For this review, take the finished solid that the model builds, in its own axes (mm). A direction names the side the tool comes from. Give positions to 0.01 mm unless a question says otherwise; leave off trailing zeros. Loops run counter-clockwise (first coordinate to the right, second up) from the corner with the lowest first, then second, coordinate; pieces in that order, holes last. Notation, with made-up numbers: (82.5, -17.75) -> (132.5, -17.75) arc R30 cw to (132.5, 12.25) -> close; hole circle Ø11 at (46, 56.25). An arc over 180 degrees is marked (long way). Write each question's results on one line, items separated by ' | '. Start each with the question number.
```python
from build123d import *

# Parameters (mm, degrees)
SKETCH103_R           = 15
SKETCH103_R_2         = 8
PAD055_DEPTH          = 8.5
POCKET033_DEPTH       = 95.040009
POLARPATTERN024_COUNT = 4
POCKET034_DEPTH       = 2
POLARPATTERN025_COUNT = 4
SKETCH108_R           = 1
POCKET035_DEPTH       = 8.501


with BuildPart() as part:
    # Sketch103 → Pad055 (new body)
    with BuildSketch(Plane.YZ):
        Circle(SKETCH103_R)
        Circle(SKETCH103_R_2, mode=Mode.SUBTRACT)
    extrude(amount=-PAD055_DEPTH)

    # Sketch107 (on Face3 of Pad055) → Pocket033 (cut, through all)
    with BuildSketch(Plane.YZ):
        with BuildLine():
            ThreePointArc((4.120305, 6.857338), (6.382423, 7.966433), (4.442476, 9.573877))
            ThreePointArc((4.851745, 12.86394), (2.086453, 11.537443), (4.442476, 9.573877))
            ThreePointArc((12.86394, 4.851745), (9.721636, 9.721636), (4.851745, 12.86394))
            ThreePointArc((9.573874, 4.442468), (11.537447, 2.086454), (12.86394, 4.851745))
            ThreePointArc((9.573874, 4.442468), (7.966437, 6.382423), (6.857338, 4.120305))
            ThreePointArc((6.857338, 4.120305), (5.656854, 5.656854), (4.120305, 6.857338))
        make_face()
    pocket033 = extrude(amount=-POCKET033_DEPTH, mode=Mode.SUBTRACT)

    # PolarPattern024: Pocket033 ×4 about axis
    polarpattern024_axis = Axis((0, 0, 0), (1, 0, 0))
    for i in range(1, POLARPATTERN024_COUNT):
        add(pocket033.rotate(polarpattern024_axis, i * 360 / POLARPATTERN024_COUNT), mode=Mode.SUBTRACT)

    # Sketch105 (on ShapeBinder) → Pocket034 (cut)
    with BuildSketch(Plane(origin=(-8.5, 0, 0), x_dir=(0, -1, 0), z_dir=(-1, 0, 0))):
        with BuildLine():
            ThreePointArc((2.107476, 12.131304), (1.313608, 13.264776), (0, 13.7))
            Line((0, 13.7), (0, 0))
            Line((0, 0), (13.7, 0))
            ThreePointArc((13.7, 0), (13.264776, 1.313608), (12.131304, 2.107476))
            Line((7.14341, 3.601623), (12.131304, 2.107476))
            ThreePointArc((7.14341, 3.601623), (5.656854, 5.656854), (3.601623, 7.14341))
            Line((2.107476, 12.131304), (3.601623, 7.14341))
        make_face()
    pocket034 = extrude(amount=-POCKET034_DEPTH, mode=Mode.SUBTRACT)

    # PolarPattern025: Pocket034 ×4 about axis
    polarpattern025_axis = Axis((-8.5, 0, 0), (-1, 0, 0))
    for i in range(1, POLARPATTERN025_COUNT):
        add(pocket034.rotate(polarpattern025_axis, i * 360 / POLARPATTERN025_COUNT), mode=Mode.SUBTRACT)

    # Sketch108 (on ShapeBinder) → Pocket035 (cut, through all)
    with BuildSketch(Plane(origin=(-8.5, 0, 0), x_dir=(0, -1, 0), z_dir=(-1, 0, 0))):
        with Locations((0, 11.5)):
            Circle(SKETCH108_R)
        with Locations((11.5, 0)):
            Circle(SKETCH108_R)
        with Locations((0, -11.5)):
            Circle(SKETCH108_R)
        with Locations((-11.5, 0)):
            Circle(SKETCH108_R)
    extrude(amount=-POCKET035_DEPTH, mode=Mode.SUBTRACT)


with BuildPart() as part_1:
    # Body038 placement: moved
    add(part.part.moved(Location((18.5, 0, 0))))


solid = part_1.part
```
1. We need section A-A (y = 11). Write out the cut boundary in (x, z).
2. Machinability: for faces 1 (the flat face through (10.99, -3.19, 8.52)), 2 (the cylindrical face through (14.31, 9.664, -9.779)), 3 (the flat face through (10, -5, 8)), which of the approach directions +Z, -Z, +X, -X, +Y, -Y give a long, thin tool a straight path to every point of the face, cutting with its end or side? Answer none if there is none.
3. We need section C-C (x = 15.75). Count the separate pieces of the cut face and the enclosed holes in it, plus the area to 3 significant figures.
4. We need section B-B (z = 11.5). Write out the cut boundary in (x, y), plus the area to 3 significant figures.
5. Wall thickness on L1, parallel to Z at x = 16, y = 0; L2, parallel to Z at x = 16.75, y = -9.75; L3, parallel to Z at x = 16.25, y = 8.5: over which ranges is each line inside the solid? List them lowest first.
6. Draft analysis for pull direction Z (two halves, no side actions). For faces 4 (the flat face through (10, -8, -5)), 5 (the flat face through (10.99, -3.2, -8.49)), state which applies: released by +Z, released by -Z, zero draft, split by the parting line, or undercut.
7. We need section D-D (z = 8.5). Write out the cut boundary in (x, y).
8. For pin 1 Ø3.5 at (y, z) = (-3.9, -11.31) entering from -X (1 decimal); pin 2 Ø4 at (x, z) = (14.5, 10.5) entering from +Y; pin 3 Ø1 at (x, y) = (11.5, 5) entering from -Z; pin 4 Ø4 at (x, z) = (13, 4.5) entering from +Y, all flat-tipped, find the tip position at first contact; note any pin that passes through.
Response:
1) outline: (10, -10.2) -> (18.5, -10.2) -> (18.5, -8.25) -> (10, -8.25) -> close; (10, 8.25) -> (18.5, 8.25) -> (18.5, 10.2) -> (10, 10.2) -> close; (12, -2.1) -> (18.5, -2.1) -> (18.5, -0.87) -> (12, -0.87) -> close; (12, 0.87) -> (18.5, 0.87) -> (18.5, 2.1) -> (12, 2.1) -> close
2) face 1: -X | face 2: +X, -X | face 3: +Z, -Z, -X, +Y, -Y
3) separate pieces: 1 | enclosed holes: 5 | area: 293 mm2
4) outline: (10, -9.63) -> (18.5, -9.63) -> (18.5, -7.53) -> (10, -7.53) -> close; (10, 7.53) -> (18.5, 7.53) -> (18.5, 9.63) -> (10, 9.63) -> close; (12, -2.08) -> (18.5, -2.08) -> (18.5, -1) -> (12, -1) -> close; (12, 1) -> (18.5, 1) -> (18.5, 2.08) -> (12, 2.08) -> close | area: 49.7 mm2
5) L1: z = -15 to -12.5, -10.5 to -8, 8 to 10.5, 12.5 to 15 | L2: z = -11.4 to -9.69, -2.96 to 2.96, 9.69 to 11.4 | L3: z = -12.36 to -10.81, -6.35 to 6.35, 10.81 to 12.36
6) face 4: zero draft | face 5: undercut
7) outline: (10, -12.36) -> (18.5, -12.36) -> (18.5, -10.81) -> (10, -10.81) -> close; (10, -6.35) -> (18.5, -6.35) -> (18.5, 6.35) -> (10, 6.35) -> (10, 3.2) -> (12, 3.2) -> (12, -3.2) -> (10, -3.2) -> close; (10, 10.81) -> (18.5, 10.81) -> (18.5, 12.36) -> (10, 12.36) -> close
8) pin 1: passes through | pin 2: stops at y = 12.36 | pin 3: stops at z = -14.31 | pin 4: stops at y = 14.79
